Input: part model. Units: mm. Frame: model coordinates. Coordinates: 2 decimals unless noted, no trailing zeros. Order: outer loops, then holes, each group sorted by start corner. A loop starts at its lowest first (then second) coordinate and runs counter-clockwise, first axis right, second up.
Autodesk Inventor part; units mm, degrees
ref_plane "YZ Plane" through (0, 0, 0) normal (1, 0, 0) x (0, 1, 0)
ref_plane "XZ Plane" through (0, 0, 0) normal (0, 1, 0) x (-1, 0, 0)
ref_plane "XY Plane" through (0, 0, 0) normal (0, 0, 1) x (1, 0, 0)
sketch "Sketch1" plane through (0, 0, 0) normal (0, 0, 1) x (1, 0, 0)
  circle A0 centre (0, 0) radius 11.43
  circle A1 centre (0, 0) radius 6.7469
  dimension "d0" = 22.86
  dimension "d1" = 13.4938
extrude "Extrusion1" add sketch "Sketch1" along normal mid plane 9.525
chamfer "Chamfer1" distance 0.4 angle 45 4 edges at (-11.43, 0, 4.7625) (-11.43, 0, -4.7625) (-6.7469, 0, 4.7625) (-6.7469, 0, -4.7625)
sketch "Sketch2" plane through (0, 0, 0) normal (1, 0, 0) x (0, 1, 0)
  point P0 (0, 0)
properties part number "3d printed nut" material "ABS Plastic"
Item 1: Pin query (flat end, axial travel): pin 1 Ø4 at (x, z) = (3, 1.5) entering from +Y; pin 2 Ø5 at (x, y) = (2.5, 2) entering from -Z. Return the tip coordinate at first contact, or that it passes through.
Response values:
pin 1: stops at y = 11.39
pin 2: passes through
Item 2: Cut plane C-C on z = -1.5. Return loops of the section in (x, y), then the cut area to 3 significant figures.
Response values:
outline: circle Ø22.86 at (0, 0); hole circle Ø13.49 at (0, 0)
area: 267 mm2
Item 3: Cut plane A-A on y = 0. Return loops of the section in (x, z).
Response values:
outline: (-11.43, -4.36) - (-11.03, -4.76) - (-7.15, -4.76) - (-6.75, -4.36) - (-6.75, 4.36) - (-7.15, 4.76) - (-11.03, 4.76) - (-11.43, 4.36) - close; (6.75, -4.36) - (7.15, -4.76) - (11.03, -4.76) - (11.43, -4.36) - (11.43, 4.36) - (11.03, 4.76) - (7.15, 4.76) - (6.75, 4.36) - close
Item 4: Ray query, probe 1 along Y at (x, z) = (0, 2.5); probe 2 along X at (y, z) = (3.75, -3.5); probe 3 along X at (y, z) = (4, 4). Return the intervals inside material, ascending.
Response values:
probe 1: y = -11.43 to -6.75, 6.75 to 11.43
probe 2: x = -10.8 to -5.61, 5.61 to 10.8
probe 3: x = -10.71 to -5.43, 5.43 to 10.71
Item 5: Draft query along Y for faces 1 (the face through (10.902, -3.433, -0.061)), 2 (the face through (6.435, -2.027, -0.061)), 3 (the face through (2.3, -7.2, -4.762)). Return one class per face: pulls with the +Y half, pulls with the -Y half, needs draft (parallel to the pull), parting line crosses it, or undercut.
Response values:
face 1: parting line crosses it
face 2: undercut
face 3: needs draft
